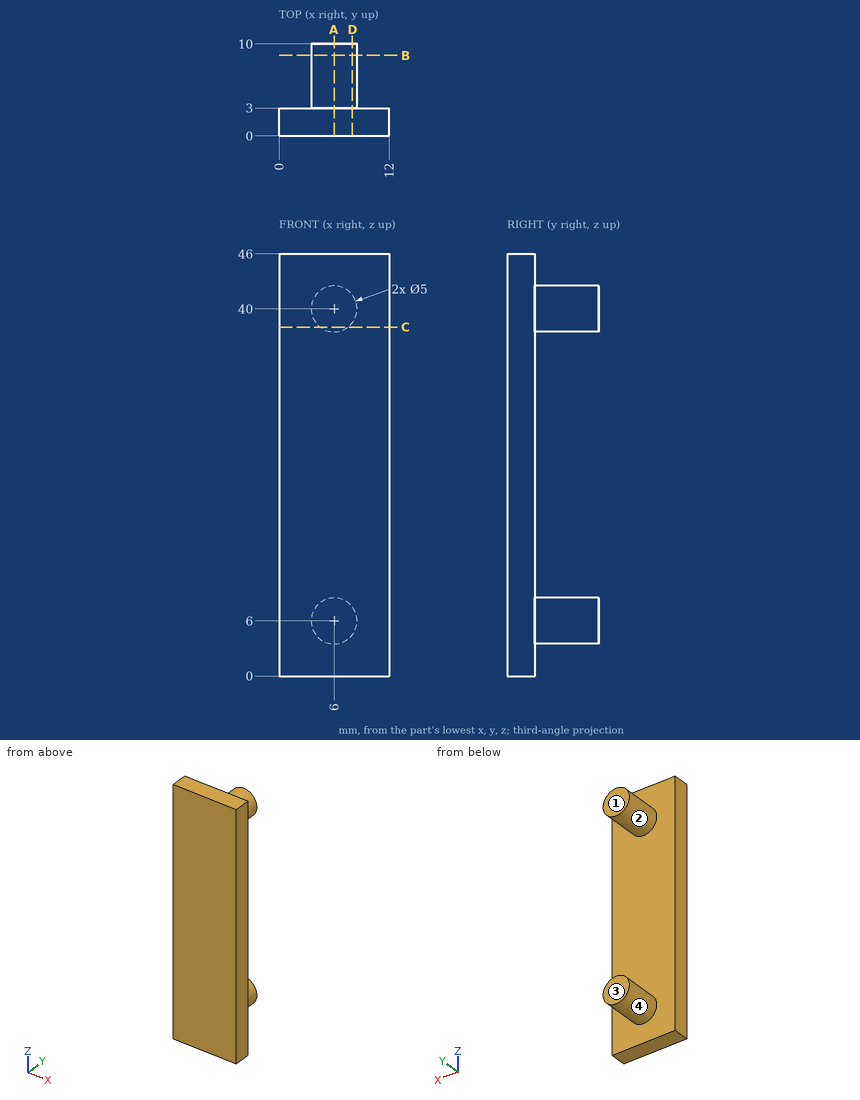
For this review, use the dimensioned drawing (mm, ordinates from the lowest corner) and the shaded views. A direction names the side the tool comes from. Give positions to 0.01 mm unless a question says otherwise; leave off trailing zeros. Order: outer loops, then holes, each group sorted by start corner. A loop starts at its lowest first (then second) coordinate and runs counter-clockwise, first axis right, second up.
1. Mouldability with a two-part tool opening along Z and no side actions: class the marked faces 1 and 2 as +Z half, -Z half, draft (parallel to the pull), parting line (faces both ways), or undercut.
Solution:
face 1: draft
face 2: undercut
2. Add section B-B, the plane y = 8.75. State the section outline as (x, z) points.
Solution:
outline: circle Ø5 at (6, 6); circle Ø5 at (6, 40)
3. For pin 1 Ø1.5 at (x, y) = (4, 1) entering from -Z; pin 2 Ø1 at (x, y) = (8.5, 7) entering from +Z, all flat-tipped, find the tip position at first contact; note any pin that passes through.
Solution:
pin 1: stops at z = 0
pin 2: stops at z = 41.5
4. To check wall thickness, follow L1, parallel to Y at x = 2.5, z = 14; L2, parallel to Z at x = 4.5, y = 6.75; L3, parallel to Z at x = 5, y = 4.75. State the ranges of each line that lie inside material, in increasing order.
Solution:
L1: y = 0 to 3
L2: z = 4 to 8, 38 to 42
L3: z = 3.71 to 8.29, 37.71 to 42.29
5. Add section D-D, the plane x = 8. State the section outline as (y, z) points, then the cut area to 3 significant figures.
Solution:
outline: (0, 0) - (3, 0) - (3, 4.5) - (10, 4.5) - (10, 7.5) - (3, 7.5) - (3, 38.5) - (10, 38.5) - (10, 41.5) - (3, 41.5) - (3, 46) - (0, 46) - close
area: 180 mm2
6. Tool access review of the marked faces 3 and 4: name each direction out of +Z, -Z, +X, -X, +Y, -Y from which nothing blocks a thin tool from reaching the whole face with its end or side.
Solution:
face 3: +Z, -Z, +X, -X, +Y
face 4: +Y
7. Add section A-A, the plane x = 6. State the section outline as (y, z) points.
Solution:
outline: (0, 0) - (3, 0) - (3, 3.5) - (10, 3.5) - (10, 8.5) - (3, 8.5) - (3, 37.5) - (10, 37.5) - (10, 42.5) - (3, 42.5) - (3, 46) - (0, 46) - close
8. Add section C-C, the plane z = 38. State the section outline as (x, y) points.
Solution:
outline: (0, 0) - (12, 0) - (12, 3) - (7.5, 3) - (7.5, 10) - (4.5, 10) - (4.5, 3) - (0, 3) - close
